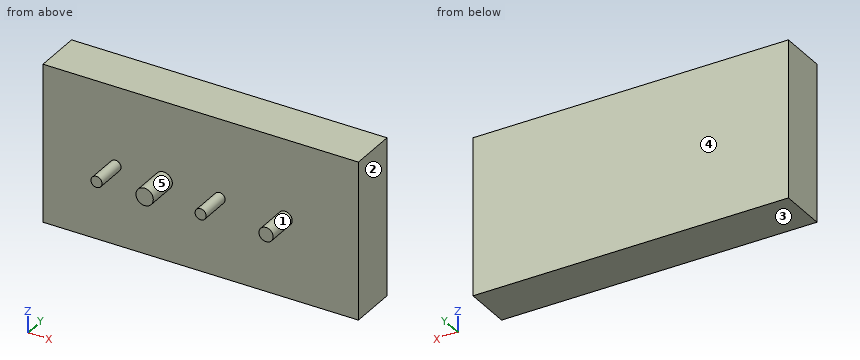
```python
from build123d import *

# Parameters (mm, degrees)
F0_W     = 100
F0_H     = 50
F1_DEPTH = 15
F2_R     = 1.75
F3_DEPTH = 10
F4_R     = 2.75
F5_DEPTH = 10
F6_R     = 1.75
F7_DEPTH = 10
F8_R     = 2.25
F9_DEPTH = 10


with BuildPart() as f1:
    # F0 (on Front) → F1 (new body)
    with BuildSketch(Plane.XZ):
        Rectangle(F0_W, F0_H)
    extrude(amount=F1_DEPTH)

    # F2 (on face) → F3 (join)
    with BuildSketch(Plane.XZ.offset(15)):
        with Locations((-27, 0)):
            Circle(F2_R)
    extrude(amount=F3_DEPTH)

    # F4 (on face) → F5 (join)
    with BuildSketch(Plane.XZ.offset(15)):
        with Locations((-11.75, 0)):
            Circle(F4_R)
    extrude(amount=F5_DEPTH)

    # F6 (on face) → F7 (join)
    with BuildSketch(Plane.XZ.offset(15)):
        with Locations((6, 0)):
            Circle(F6_R)
    extrude(amount=F7_DEPTH)

    # F8 (on face) → F9 (join)
    with BuildSketch(Plane.XZ.offset(15)):
        with Locations((26.75, 0)):
            Circle(F8_R)
    extrude(amount=F9_DEPTH)


solid = f1.part
```
For this review, take the finished solid that the model builds, in its own axes (mm). Face numbers are marked on the shaded views. A direction names the side the tool comes from. Round coordinates to 2 decimals unless told otherwise and drop trailing zeros. Order: outer loops, then holes, each group sorted by start corner. A loop starts at its lowest first (then second) coordinate and runs counter-clockwise, first axis right, second up.
Q1. We need section C-C, the plane z = 0. Give the boundary of the cut face in (x, y).
Findings below:
outline: (-50, -15) - (-28.75, -15) - (-28.75, -25) - (-25.25, -25) - (-25.25, -15) - (-14.5, -15) - (-14.5, -25) - (-9, -25) - (-9, -15) - (4.25, -15) - (4.25, -25) - (7.75, -25) - (7.75, -15) - (24.5, -15) - (24.5, -25) - (29, -25) - (29, -15) - (50, -15) - (50, 0) - (-50, 0) - close
Q2. Mouldability with a two-part tool opening along X and no side actions: class the marked faces 1, 2 and 3 as pulls with the +X half, pulls with the -X half, needs draft (parallel to the pull), parting line crosses it, or undercut.
Findings below:
face 1: undercut
face 2: pulls with the +X half
face 3: needs draft
Q3. We need section D-D, the plane x = 26.75. Give the boundary of the cut face in (y, z), plus the area to 3 significant figures.
Findings below:
outline: (-25, -2.25) - (-15, -2.25) - (-15, -25) - (0, -25) - (0, 25) - (-15, 25) - (-15, 2.25) - (-25, 2.25) - close
area: 795 mm2
Q4. Machinability: for the marked faces 4 and 5, which of the approach directions +Z, -Z, +X, -X, +Y, -Y give a long, thin tool a straight path to every point of the face, cutting with its end or side? Answer none if there is none.
Findings below:
face 4: +Z, -Z, +X, -X, +Y
face 5: -Y
Q5. Insertion check: P1, Ø4, axis at x = -4.5, z = 8, coming from the -Y side; P2, Ø6, axis at x = -23, y = -21.5, coming from the +Z side. Each pin has a flat end and moves straight along its axis. Give the tip position at first contact, or say it passes through.
Findings below:
P1: stops at y = -15
P2: stops at z = 1.44
Q6. We need section A-A, the plane x = -11.75. Give the boundary of the cut face in (y, z).
Findings below:
outline: (-25, -2.75) - (-15, -2.75) - (-15, -25) - (0, -25) - (0, 25) - (-15, 25) - (-15, 2.75) - (-25, 2.75) - close
Q7. Wall thickness on line 1 (Y direction, x = 19, z = -19.5): over which ranges is the line inside the solid? List them lowest first.
Findings below:
line 1: y = -15 to 0
Q8. We need section B-B, the plane y = -17.75. Give the boundary of the cut face in (x, z).
Findings below:
outline: circle Ø3.5 at (-27, 0); circle Ø5.5 at (-11.75, 0); circle Ø3.5 at (6, 0); circle Ø4.5 at (26.75, 0)
